Check sheet for the modelled part. Datum: model origin and axes. Units: mm. A direction names the side the tool comes from. Give positions to 0.01 mm unless a question says otherwise; leave off trailing zeros. Write each loop counter-clockwise with the first axis right and the second up, starting at its lowest first coordinate (ties: lowest second). Pieces come first, ordered by that corner, then holes. Notation, with made-up numbers: M -28,47 L 4,47 A32 ccw 4,78 Z; hole C 54,-0.5 d1. An arc over 180 degrees is marked long. Write item = value, one per line. Start each with the question number.
1) Sectioned sample at A-A, the plane x = 7.5. Record the cut outline in (y, z).
2) Sectioned sample at B-B, the plane z = 0.75. Record the cut outline in (x, y).
3) Set-up check for faces 5 (the face through (0, 2.5, 0)), 6 (the face through (0.07, 0.246, 4.986)), 7 (the face through (-5, 1, 6)), 8 (the face through (5, 1, 6)), 9 (the face through (-15, 1, 0)): record each of +Z, -Z, +X, -X, +Y, -Y from which the full face is reachable in a straight line by a thin tool's end or side.
4) Sectioned sample at D-D, the plane x = 3. Record the cut outline in (y, z), then the cut area to 3 significant figures.
5) Draft check along Y on faces 1 (the face through (-10, 1, 4)), 2 (the face through (0, 0, 0)), 3 (the face through (0.07, 3.867, 7.46)), 4 (the face through (0.07, 2.55, 7.25)). Enter one of: pulls with the +Y half, pulls with the -Y half, needs draft (parallel to the pull), parting line crosses it, or undercut.
6) Scan lines: L1, parallel to X at y = 1.4, z = 0; L2, parallel to Z at x = 2, y = 2.6; L3, parallel to X at y = 1.45, z = 2.25. Record each from-to range of solid material in increasing order.
7) Gauge pin test, flat ends, axial feed: pin 1 (0.8 mm diameter, centred on x = -9, y = 1.5, fed in from +Z); pin 2 (4 mm diameter, centred on x = 7.5, z = 0, fed in from -Y); pin 3 (1.2 mm diameter, centred on y = 1.5, z = 6.5, fed in from +X); pin 4 (2 mm diameter, centred on y = 2, z = 5.5, fed in from -X). Record the tip position at first contact, or that the pin passes through.
8) Sectioned sample at C-C, the plane y = 3.45. Record the cut outline in (x, z).
from build123d import *

# Parameters (mm, degrees)
SKETCH1_W                       = 30
SKETCH1_H                       = 8
SKETCH1_R                       = 2.5
BOSS_EXTRUDE1_DEPTH             = 2.5
BOSS_EXTRUDE2_REACH             = 17
SKETCH2_R                       = 1.25
BOSS_EXTRUDE2_DIRECTION_2_REACH = 17
SKETCH4_W                       = 10
SKETCH4_H                       = 4
CUT_EXTRUDE2_DEPTH              = 5.5


with BuildPart() as part:
    # Sketch1 → Boss-Extrude1 (new body)
    with BuildSketch(Plane(origin=(0, 0, 0), x_dir=(1, 0, 0), z_dir=(0, 1, 0))):
        Rectangle(SKETCH1_W, SKETCH1_H)
        with Locations((-7.5, 0)):
            Circle(SKETCH1_R, mode=Mode.SUBTRACT)
        with Locations((7.5, 0)):
            Circle(SKETCH1_R, mode=Mode.SUBTRACT)
    extrude(amount=BOSS_EXTRUDE1_DEPTH)

    # Boss-Extrude2: up to this face of the body (flat: up to its plane)
    boss_extrude2_end = Plane(part.part.faces().sort_by_distance((15, 1.25, 0))[0])
    # Sketch2 → Boss-Extrude2 (add, up to the picked face)
    with BuildSketch(Plane(origin=(0, 0, 0), x_dir=(0, 0, -1), z_dir=(1, 0, 0)), mode=Mode.PRIVATE) as boss_extrude2_sk1:
        with BuildLine():
            Line((-4, 2.5), (-4, 0))
            Line((-4, 0), (-6, 0.5))
            ThreePointArc((-6, 0.5), (-7.414213562, 3.914213562), (-4, 2.5))
        make_face()
        with Locations((-6, 2.5)):
            Circle(SKETCH2_R, mode=Mode.SUBTRACT)
    boss_extrude2_tool1 = split(extrude(boss_extrude2_sk1.sketch, amount=BOSS_EXTRUDE2_REACH, mode=Mode.PRIVATE), bisect_by=boss_extrude2_end, keep=Keep.BOTH, mode=Mode.PRIVATE)
    add(boss_extrude2_tool1.solids().sort_by_distance((0, 1.25, 4.060208))[0])

    # Boss-Extrude2 direction 2: up to this face of the body (flat: up to its plane)
    boss_extrude2_direction_2_end = Plane(part.part.faces().sort_by_distance((-15, 1.25, 0))[0])
    # Sketch2 → Boss-Extrude2 direction 2 (add, up to the picked face)
    with BuildSketch(Plane(origin=(0, 0, 0), x_dir=(0, 0, -1), z_dir=(1, 0, 0)), mode=Mode.PRIVATE) as boss_extrude2_direction_2_sk1:
        with BuildLine():
            Line((-4, 2.5), (-4, 0))
            Line((-4, 0), (-6, 0.5))
            ThreePointArc((-6, 0.5), (-7.414213562, 3.914213562), (-4, 2.5))
        make_face()
        with Locations((-6, 2.5)):
            Circle(SKETCH2_R, mode=Mode.SUBTRACT)
    boss_extrude2_direction_2_tool1 = split(extrude(boss_extrude2_direction_2_sk1.sketch, amount=-BOSS_EXTRUDE2_DIRECTION_2_REACH, mode=Mode.PRIVATE), bisect_by=boss_extrude2_direction_2_end, keep=Keep.BOTH, mode=Mode.PRIVATE)
    add(boss_extrude2_direction_2_tool1.solids().sort_by_distance((0, 1.25, 4.060208))[0])

    # Sketch4 → Cut-Extrude2 (cut, through all)
    with BuildSketch(Plane(origin=(0, 0, 0), x_dir=(1, 0, 0), z_dir=(0, 1, 0))):
        with Locations((-10, -6)):
            Rectangle(SKETCH4_W, SKETCH4_H)
        with Locations((10, -6)):
            Rectangle(SKETCH4_W, SKETCH4_H)
    extrude(amount=CUT_EXTRUDE2_DEPTH, mode=Mode.SUBTRACT)


solid = part.part
Data:
q1.outline = M 0,-4 L 2.5,-4 L 2.5,-2.5 L 0,-2.5 Z; M 0,2.5 L 2.5,2.5 L 2.5,4 L 0,4 Z
q2.outline = M -15,0 L -9.88,0 L -9.88,2.5 L -15,2.5 Z; M -5.12,0 L 5.12,0 L 5.12,2.5 L -5.12,2.5 Z; M 9.88,0 L 15,0 L 15,2.5 L 9.88,2.5 Z
q3.face_5 = -Z, +X, -X, +Y
q3.face_6 = +Z, +X, -X, -Y
q3.face_7 = +Z, -X, +Y, -Y
q3.face_8 = +Z, +X, +Y, -Y
q3.face_9 = +Z, -Z, -X, +Y, -Y
q4.outline = M 0,-4 L 2.5,-4 L 2.5,4 A2 ccw long 0.5,6 L 0,4 Z; hole C 2.5,6 d2.5
q4.area = 29.0 mm2
q5.face_1 = needs draft
q5.face_2 = pulls with the -Y half
q5.face_3 = parting line crosses it
q5.face_4 = undercut
q6.L1 = -15 to -10, -5 to 5, 10 to 15
q6.L2 = 4 to 4.75, 7.25 to 8
q6.L3 = -15 to -8.59, -6.41 to 6.41, 8.59 to 15
q7.pin_1 = 4
q7.pin_2 = through
q7.pin_3 = 5
q7.pin_4 = -5
q8.outline = M -5,4.24 L 5,4.24 L 5,5.19 L -5,5.19 Z; M -5,6.81 L 5,6.81 L 5,7.76 L -5,7.76 Z
